The listing builds one solid part. Answer for the finished solid, in the listing's coordinates (mm). A direction names the side the tool comes from. Give positions to 0.01 mm unless a question says otherwise; leave off trailing zeros. Loops run counter-clockwise (first coordinate to the right, second up) from the corner with the lowest first, then second, coordinate; pieces in that order, holes last. Notation, with made-up numbers: M 76,89.5 L 118,89.5 A11 cw 118,109.5 Z; hole C -13.75,82.5 d1. An arc over 180 degrees is marked long. Return JSON: item names as keys, results as strings.
from build123d import *

# Parameters (mm, degrees)
BOSS_EXTRUDE1_DEPTH = 9
FILLET1_R           = 30
FILLET2_R           = 3
BOSS_EXTRUDE2_DEPTH = 0.1
SKETCH3_R           = 1.2
CUT_EXTRUDE1_DEPTH  = 5
SKETCH4_W           = 3.5
SKETCH4_H           = 14.5
CUT_EXTRUDE2_DEPTH  = 1.5
SKETCH5_W           = 2.5
SKETCH5_H           = 11
CUT_EXTRUDE4_DEPTH  = 1.5
FILLET3_R           = 1


with BuildPart() as part:
    # Sketch1 → Boss-Extrude1 (new body)
    with BuildSketch(Plane.XY):
        Polygon((78, -16.25), (78, 16.25), (-78, 16.25), (-78, -16.25), (-30, -16.25), (-15, -19.25), (15, -19.25), (30, -16.25), align=None)
    extrude(amount=BOSS_EXTRUDE1_DEPTH)

    # Fillet1
    fillet1_edges = [part.edges().sort_by_distance(p)[0] for p in [
        (30, -16.25, 4.5),
        (15, -19.25, 4.5),
        (-15, -19.25, 4.5),
        (-30, -16.25, 4.5),
    ]]
    fillet(fillet1_edges, radius=FILLET1_R)

    # Fillet2
    fillet2_edges = [part.edges().sort_by_distance(p)[0] for p in [
        (-78, 16.25, 4.5),
        (78, 16.25, 4.5),
        (78, -16.25, 4.5),
        (-78, -16.25, 4.5),
    ]]
    fillet(fillet2_edges, radius=FILLET2_R)

    # Sketch2 → Boss-Extrude2 (add)
    with BuildSketch(Plane.XY.offset(9)):
        with BuildLine():
            Line((-32.970585408, -15.75), (32.970585408, -15.75))
            Line((32.970585408, -15.75), (75, -15.75))
            ThreePointArc((75, -15.75), (76.767766953, -15.017766953), (77.5, -13.25))
            Line((77.5, -13.25), (77.5, 13.25))
            ThreePointArc((77.5, 13.25), (76.767766953, 15.017766953), (75, 15.75))
            Line((75, 15.75), (-75, 15.75))
            ThreePointArc((-75, 15.75), (-76.767766953, 15.017766953), (-77.5, 13.25))
            Line((-77.5, 13.25), (-77.5, -13.25))
            ThreePointArc((-77.5, -13.25), (-76.767766953, -15.017766953), (-75, -15.75))
            Line((-75, -15.75), (-32.970585408, -15.75))
        make_face()
    extrude(amount=BOSS_EXTRUDE2_DEPTH)

    # Sketch3 → Cut-Extrude1 (cut)
    with BuildSketch(Plane.XZ.offset(19.25)):
        with Locations((-9, 4.5)):
            Circle(SKETCH3_R)
        with Locations(Location((9, 4.5, 0), (0, 0, 180))):
            Circle(SKETCH3_R)
    extrude(amount=-CUT_EXTRUDE1_DEPTH, mode=Mode.SUBTRACT)

    # Sketch4 → Cut-Extrude2 (cut)
    with BuildSketch(Plane.ZY.offset(78)):
        with Locations((5.75, -1)):
            Rectangle(SKETCH4_W, SKETCH4_H)
    extrude(amount=-CUT_EXTRUDE2_DEPTH, mode=Mode.SUBTRACT)

    # Sketch5 → Cut-Extrude4 (cut)
    with BuildSketch(Plane(origin=(78, 0, 0), x_dir=(0, 0, -1), z_dir=(1, 0, 0))):
        with Locations((-5.75, -7.25)):
            Rectangle(SKETCH5_W, SKETCH5_H)
    extrude(amount=-CUT_EXTRUDE4_DEPTH, mode=Mode.SUBTRACT)

    # Fillet3
    fillet3_edges = [part.edges().sort_by_distance(p)[0] for p in [
        (-77.25, -8.25, 4),
        (-77.25, 6.25, 4),
        (-77.25, 6.25, 7.5),
        (-77.25, -8.25, 7.5),
        (77.25, -12.75, 7),
        (77.25, -1.75, 7),
        (77.25, -1.75, 4.5),
        (77.25, -12.75, 4.5),
    ]]
    fillet(fillet3_edges, radius=FILLET3_R)


solid = part.part
(1) Straight lines are drawn through the part: line 1 along Z through (x, y) = (9, -17.6); line 2 along Y through (x, z) = (-13, 1.5); line 3 along Y through (x, z) = (47, 6.5). For each, find the intervals that lie inside material, in ascending order.
Values follow:
{"line 1": "0 to 3.3, 5.7 to 9", "line 2": "-19.23 to 16.25", "line 3": "-16.25 to 16.25"}
(2) Determine the mould class of faces 4 (the flat face through (-1, -1, 0)), 5 (the flat face through (-76.5, -1, 6)), 6 (the flat face through (54, -16.25, 4)), 7 (the cylindrical face through (77.1, 15.39, 4.56)) for opening direction Y: released by +Y, released by -Y, zero draft, split by the parting line, or undercut.
Values follow:
{"face 4": "zero draft", "face 5": "undercut", "face 6": "released by -Y", "face 7": "released by +Y"}
(3) The part is cut by section A-A (x = -61.5). Determine the outline of the cut face in (y, z).
Values follow:
{"outline": "M -16.25,0 L 16.25,0 L 16.25,9 L 15.75,9 L 15.75,9.1 L -15.75,9.1 L -15.75,9 L -16.25,9 Z"}
(4) The part is cut by section B-B (z = 1.75). Determine the outline of the cut face in (x, y), and give its area (3 significant figures).
Values follow:
{"outline": "M -78,-13.25 A3 ccw -75,-16.25 L -32.97,-16.25 A30 cw -27.09,-16.83 L -17.91,-18.67 A30 ccw -12.03,-19.25 L 12.03,-19.25 A30 ccw 17.91,-18.67 L 27.09,-16.83 A30 cw 32.97,-16.25 L 75,-16.25 A3 ccw 78,-13.25 L 78,13.25 A3 ccw 75,16.25 L -75,16.25 A3 ccw -78,13.25 Z", "area": "5,200 mm²"}
(5) Given pin 1 (0.6 mm diameter, centred on x = 77, z = 5.5, fed in from -Y); pin 2 (12 mm diameter, centred on x = -23.5, y = 3, fed in from -Z); pin 3 (4.5 mm diameter, centred on x = -48, z = 4.5, fed in from -Y); pin 4 (0.7 mm diameter, centred on x = 8.5, z = 4.5, fed in from -Y), each flat-ended and moving along its own axis, determine where each tip first touches the part or whether it passes through.
Values follow:
{"pin 1": "y = -15.72", "pin 2": "z = 0", "pin 3": "y = -16.25", "pin 4": "y = -14.25"}
(6) A tool of negligible diameter and unlimited length cuts with its end or side. For faces 1 (the flat face through (-54, -16.25, 4)), 2 (the cylindrical face through (-77.14, 15.35, 4.56)), 3 (the flat face through (76.5, -7, 6)), from which of +Z, -Z, +X, -X, +Y, -Y can it reach the whole face along a straight path? Write none if from no direction.
Values follow:
{"face 1": "+Z, -Z, -X, -Y", "face 2": "+Z, -Z, -X, +Y", "face 3": "+X"}
